Geometry check sheet. Reference: the model listing, model coordinates, mm. Face numbers are marked on the shaded views. Round coordinates to 2 decimals unless told otherwise and drop trailing zeros. Write each loop counter-clockwise with the first axis right and the second up, starting at its lowest first coordinate (ties: lowest second). Pieces come first, ordered by that corner, then holes. Notation, with made-up numbers: M -20,67.5 L 4,67.5 A14 cw 4,74.5 Z; hole C 15,31 d9. An arc over 180 degrees is marked long. Answer in a Markdown table with one row per item. Add a question column.
Autodesk Inventor part; units mm, degrees
ref_plane "Arbeitsebene1" through (0, 0, 0) normal (0, 1, 0) x (-1, 0, 0)
ref_plane "Arbeitsebene2" through (12, 0, 0) normal (1, 0, 0) x (0, 1, 0)
ref_plane "Arbeitsebene3" through (-142.5, 0, 0) normal (1, 0, 0) x (0, 1, 0)
sketch "Skizze1" plane through (0, 0, 0) normal (0, 1, 0) x (-1, 0, 0)
  arc A0 (10.3923, 6) -> (10.3923, -6) centre (0, 0) ccw
  line L0 (10.3923, 6) -> (150, 6)
  line L1 (150, 6) -> (150, -6)
  line L2 (150, -6) -> (10.3923, -6)
  line L3 (0, 0) -> (150, 0) construction
  circle A1 centre (0, 0) radius 3.75
  dimension "d0" = 24
  dimension "d1" = 12
  dimension "d2" = 7.5
  dimension "d3" = 150
extrude "Extrusion1" add sketch "Skizze1" along normal mid plane 12
ref_plane "Arbeitsebene1" through (0, 0, 0) normal (0, 1, 0) x (-1, 0, 0)
sketch "Skizze2" plane through (0, 0, 0) normal (0, 1, 0) x (-1, 0, 0)
  line L0 (150, 6) -> (150, -6)
  circle A0 centre (150, 0) radius 12
  point P0 (0, 0)
  dimension "d7" = 24
extrude "Extrusion2" add sketch "Skizze2" along normal mid plane 12
sketch "Skizze3" plane through (0, 6, 0) normal (0, 1, 0) x (1, 0, 0)
  arc A0 (-139.6077, 6) -> (-139.6077, -6) centre (-150, 0) ccw
  point P0 (0, 0)
hole "Bohrung1" at (-150, 6, 0) direction (0, -1, 0) diameter 7.5 depth 12
sketch "Skizze4" plane through (0, 6, 0) normal (0, 1, 0) x (1, 0, 0)
  line L0 (-17, 0) -> (-109, 0) construction
  line L1 (-17, 3) -> (-109, 3)
  line L2 (-109, -3) -> (-17, -3)
  arc A0 (-17, -3) -> (-17, 3) centre (-17, 0) ccw
  arc A1 (-109, 3) -> (-109, -3) centre (-109, 0) ccw
  circle A2 centre (-150, 0) radius 3.75
  point P0 (0, 0)
  point P1 (-63, 0)
  point P2 (-14, 0)
  point P3 (-112, 0)
  point P4 (-63, 3)
  dimension "d18" = 6
  dimension "d20" = 98
  dimension "d21" = 150
  dimension "d22" = 14
extrude "Extrusion3" cut sketch "Skizze4" against normal blind 4 contours A0 L2 A1 L1
mirror "Spiegeln1" about plane through (0, 0, 0) normal (0, 1, 0) of "Extrusion3"
ref_plane "Arbeitsebene2" through (12, 0, 0) normal (1, 0, 0) x (0, 1, 0)
sketch "Skizze5" plane through (12, 0, 0) normal (1, 0, 0) x (0, 1, 0)
  point P0 (0, 0)
  point P1 (0, 0)
sketch "Skizze6" plane through (-142.5, 0, 0) normal (1, 0, 0) x (0, 1, 0)
  point P0 (0, 0)
  point P1 (0, 0)
properties part number "pleuel_third" material "Nickel-Kupfer-Legierung 400"
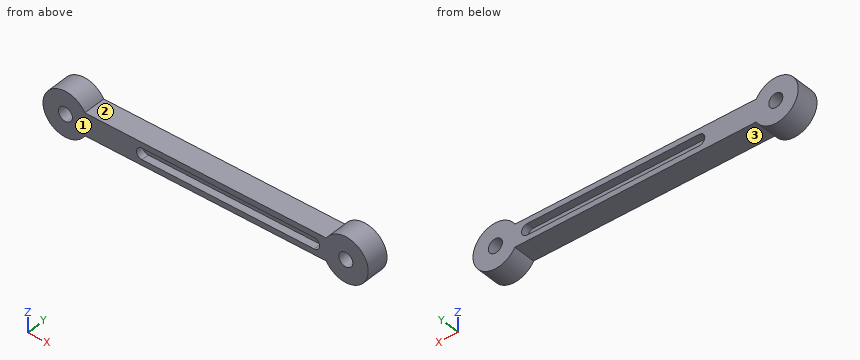
Item 1: Scan lines: probe 1 along Z at (x, y) = (-28, -2.75); probe 2 along Z at (x, y) = (-149.5, -0.5); probe 3 along X at (y, z) = (3.25, 2.5). Record each from-to range of solid material in increasing order. Write a range as from..to.
Item 2: Gauge pin test, flat ends, axial feed: pin 1 Ø1.2 at (x, y) = (-48, 3.5) entering from +Z; pin 2 Ø6.5 at (x, z) = (-77.5, -1) entering from -Y; pin 3 Ø3 at (x, y) = (-84.5, 3.5) entering from -Z; pin 4 Ø3 at (x, z) = (-58.5, 1) entering from +Y. Record the tip position at first contact, or that the pin passes through.
Item 3: Section check D-D, the plane x = -56.5. Record the boundary of the cut face in (y, z).
Item 4: Mould release check, pull along X, two halves, no side actions. Record for the marked faces 1, 2 and 3: +X half, -X half, draft (parallel to the pull), parting line (faces both ways), or undercut.
Item 5: Section check A-A, the plane x = -150. Record the boundary of the cut face in (y, z).
Item 6: Section check B-B, the plane z = 0. Record the boundary of the cut face in (x, y).
Item 7: Section check C-C, the plane y = -4.5. Record the boundary of the cut face in (x, z), and give its area (3 significant figures).
Result sheet:
| question | item | result |
|---|---|---|
| 1 | probe 1 | z = -6..-3, 3..6 |
| 1 | probe 2 | z = -11.99..-3.72, 3.72..11.99 |
| 1 | probe 3 | x = -161.74..-152.8, -147.2..-110.66, -15.34..-2.8, 2.8..11.74 |
| 2 | pin 1 | stops at z = 6 |
| 2 | pin 2 | stops at y = -6 |
| 2 | pin 3 | stops at z = -6 |
| 2 | pin 4 | stops at y = 2 |
| 3 | outline | M -6,-6 L 6,-6 L 6,-3 L 2,-3 L 2,3 L 6,3 L 6,6 L -6,6 L -6,3 L -2,3 L -2,-3 L -6,-3 Z |
| 4 | face 1 | draft |
| 4 | face 2 | undercut |
| 4 | face 3 | undercut |
| 5 | outline | M -6,-12 L 6,-12 L 6,-3.75 L -6,-3.75 Z; M -6,3.75 L 6,3.75 L 6,12 L -6,12 Z |
| 6 | outline | M -162,-6 L -153.75,-6 L -153.75,6 L -162,6 Z; M -146.25,-6 L -112,-6 L -112,-2 L -14,-2 L -14,-6 L -3.75,-6 L -3.75,6 L -14,6 L -14,2 L -112,2 L -112,6 L -146.25,6 Z; M 3.75,-6 L 12,-6 L 12,6 L 3.75,6 Z |
| 7 | outline | M -139.61,-6 L -10.39,-6 A12 ccw long -10.39,6 L -139.61,6 A12 ccw long Z; hole C -150,0 d7.5; hole M -109,-3 L -17,-3 A3 ccw -17,3 L -109,3 A3 ccw Z; hole C 0,0 d7.5 |
| 7 | area | 1,760 mm^2 |
